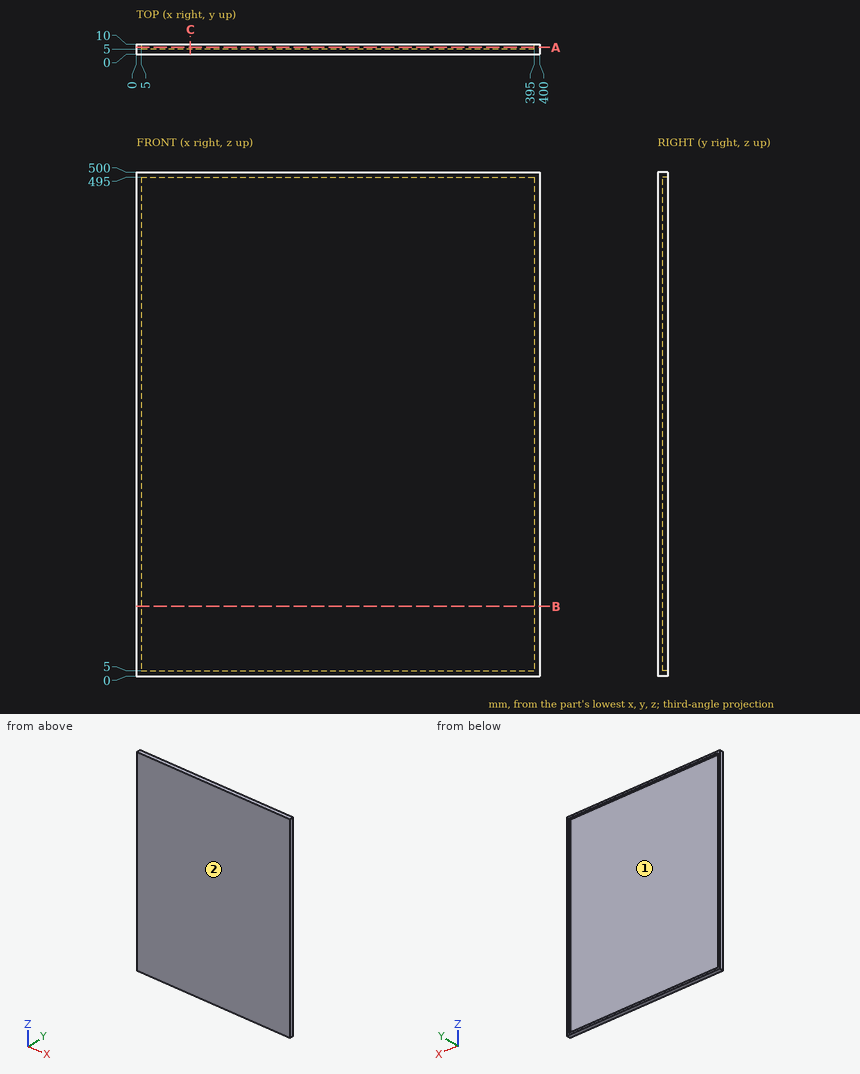
For this review, use the dimensioned drawing (mm, ordinates from the lowest corner) and the shaded views. Round coordinates to 2 decimals unless told otherwise and drop trailing zeros. Write each loop counter-clockwise with the first axis right and the second up, starting at its lowest first coordinate (ties: lowest second). Pieces come first, ordered by that corner, then holes. Notation, with made-up numbers: (67, -25.75) -> (92, -25.75) arc R15 ccw to (92, -5.75) -> close; hole circle Ø4 at (17.5, -29.5). An arc over 180 degrees is marked (long way). Use one line per item in the form item = value.
Q1. Consider section C-C (x = 53.5). State the section outline as (y, z) points, then the cut area to 3 significant figures.
Resolved:
outline = (0, 0) -> (10, 0) -> (10, 5) -> (5, 5) -> (5, 495) -> (10, 495) -> (10, 500) -> (0, 500) -> close
area = 2,550 mm²
Q2. Consider section B-B (z = 69). State the section outline as (x, y) points, then the cut area to 3 significant figures.
Resolved:
outline = (0, 0) -> (400, 0) -> (400, 10) -> (395, 10) -> (395, 5) -> (5, 5) -> (5, 10) -> (0, 10) -> close
area = 2,050 mm²
Q3. Consider section A-A (y = 6.75). State the section outline as (x, z) points.
Resolved:
outline = (0, 0) -> (400, 0) -> (400, 500) -> (0, 500) -> close; hole (5, 5) -> (395, 5) -> (395, 495) -> (5, 495) -> close
Q4. The part is to be moulded in two halves that separate along Z. For the marked faces 1 and 2, say which applies: released by +Z, released by -Z, zero draft, split by the parting line, or undercut.
Resolved:
face_1 = undercut
face_2 = zero draft
Q5. Clearance check with a flat-ended pin moving along its axis: pin 1 Ø4 at (y, z) = (8, 112) entering from -X. State where the tip first meets the part, or that it passes through.
Resolved:
pin_1 = 0
Q6. To check wall thickness, follow probe 1 along X at (y, z) = (6, 409); probe 2 along Z at (x, y) = (230.5, 7.75); probe 3 along Y at (x, z) = (333.5, 69). State the ranges of each line that lie inside material, in increasing order. Write a range as from..to.
Resolved:
probe_1 = 0..5, 395..400
probe_2 = 0..5, 495..500
probe_3 = 0..5
